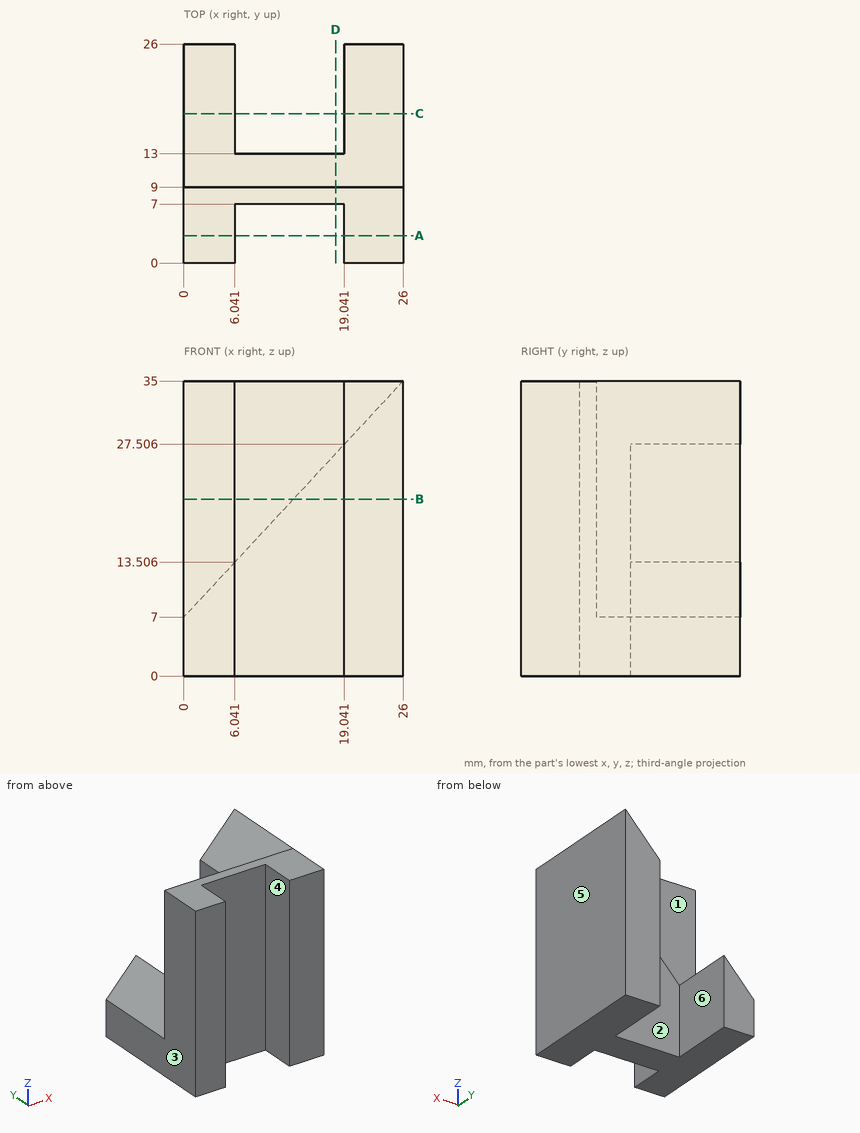
Can you work these out from the drawing? Everything is in mm from the part's minimum corner. A direction names the side the tool comes from. Round coordinates to 2 decimals unless told otherwise and drop trailing zeros. Write each loop counter-clockwise with the first axis right and the second up, starting at its lowest first coordinate (ties: lowest second). Pieces come first, ordered by that corner, then holes.
1. Will these pins go through, and if not, where does the flat tip stop? pin 1 Ø6.5 at (x, z) = (13, 12.5) entering from +Y; pin 2 Ø10.5 at (x, z) = (12, 13.5) entering from -Y; pin 3 Ø10.5 at (y, z) = (18.5, 14) entering from -X (1 decimal).
2. Suppose I cut it at A-A (y = 3.25). List the corners of the cut face in (x, z) for me, and give its area (3 significant figures).
3. Suppose I cut it at B-B (z = 21). List the corners of the cut face in (x, y) for me.
4. I need wall thicknesses on L1, parallel to X at y = 6.25, z = 13; L2, parallel to Y at x = 8, z = 6; L3, parallel to Y at x = 2.5, z = 11. Which ranges of each line are inside material? Lowest first, please.
5. For the marked faces 4, 5 and 6, which set-ups out of +Z, -Z, +X, -X, +Y, -Y let a thin tool reach every point of the face, with its end or its side?
6. Suppose I cut it at D-D (x = 18). List the corners of the cut face in (y, z) for me.
7. Suppose I cut it at C-C (y = 17.75). List the corners of the cut face in (x, z) for me.
8. If we mould it in two halves opening along X, with no side actions, what happens to the marked faces 1, 2 and 3? For each: released by +X, released by -X, zero draft, split by the parting line, or undercut.
Answer sheet:
1. pin 1: stops at y = 13
1. pin 2: stops at y = 7
1. pin 3: stops at x = 1.6
2. outline: (0, 0) - (6.04, 0) - (6.04, 35) - (0, 35) - close; (19.04, 0) - (26, 0) - (26, 35) - (19.04, 35) - close
2. area: 455 mm2
3. outline: (0, 0) - (6.04, 0) - (6.04, 7) - (19.04, 7) - (19.04, 0) - (26, 0) - (26, 26) - (19.04, 26) - (19.04, 13) - (13, 13) - (13, 9) - (0, 9) - close
4. L1: x = 0 to 6.04, 19.04 to 26
4. L2: y = 7 to 13
4. L3: y = 0 to 9
5. face 4: +Z, -Z, -Y
5. face 5: +Z, -Z, +X, +Y, -Y
5. face 6: +Z, -Z, +Y
6. outline: (7, 0) - (13, 0) - (13, 26.38) - (9, 26.38) - (9, 35) - (7, 35) - close
7. outline: (0, 0) - (6.04, 0) - (6.04, 13.51) - (0, 7) - close; (19.04, 0) - (26, 0) - (26, 35) - (19.04, 27.51) - close
8. face 1: zero draft
8. face 2: undercut
8. face 3: released by -X
